Job drawing, mm, ordinate dimensions from the low corner. One solid piece. A direction names the side the tool comes from. Give positions to 0.01 mm unless a question says otherwise; leave off trailing zeros. Write each loop counter-clockwise with the first axis right and the second up, starting at its lowest first coordinate (ties: lowest second). Pieces come first, ordered by that corner, then holes. Notation, with made-up numbers: (66.5, -39.5) - (111.5, -39.5) arc R35 ccw to (111.5, -2.5) - close; hole circle Ø4 at (-32, 32). An arc over 180 degrees is marked (long way). Put each result on its own line as item: value. Start each with the question number.
1. Drop a flat-ended pin along its axis: pin 1 (1.5 mm diameter, centred on x = 2.5, z = 2.5, fed in from +Y). Give the stop position or say it passes through.
2. Cut at D-D on x = 0.6. List the corners of the cut face in (y, z).
3. Cut at A-A on y = 11.25. List the corners of the cut face in (x, z) (1 decimal).
4. Cut at C-C on x = 2.3. List the corners of the cut face in (y, z), and give its area (3 significant figures).
5. Tool access for the marked faces 1 and 2: list every direction of +Z, -Z, +X, -X, +Y, -Y with a clear straight run to the whole face (end or side of a thin tool).
6. Wall check: line 1 (Y direction, x = 0.25, z = 6.75); line 2 (X direction, y = 10, z = 11.25); line 3 (Z direction, x = 1, y = 7.25) (1 decimal). Give the ranges that are in metal, low to high.
7. Cut at B-B on z = 3.75. List the corners of the cut face in (x, y).
8. Mould opens along Z. For the marked faces 3, 4 and 5 say: +Z half, -Z half, draft (parallel to the pull), parting line (faces both ways), or undercut.
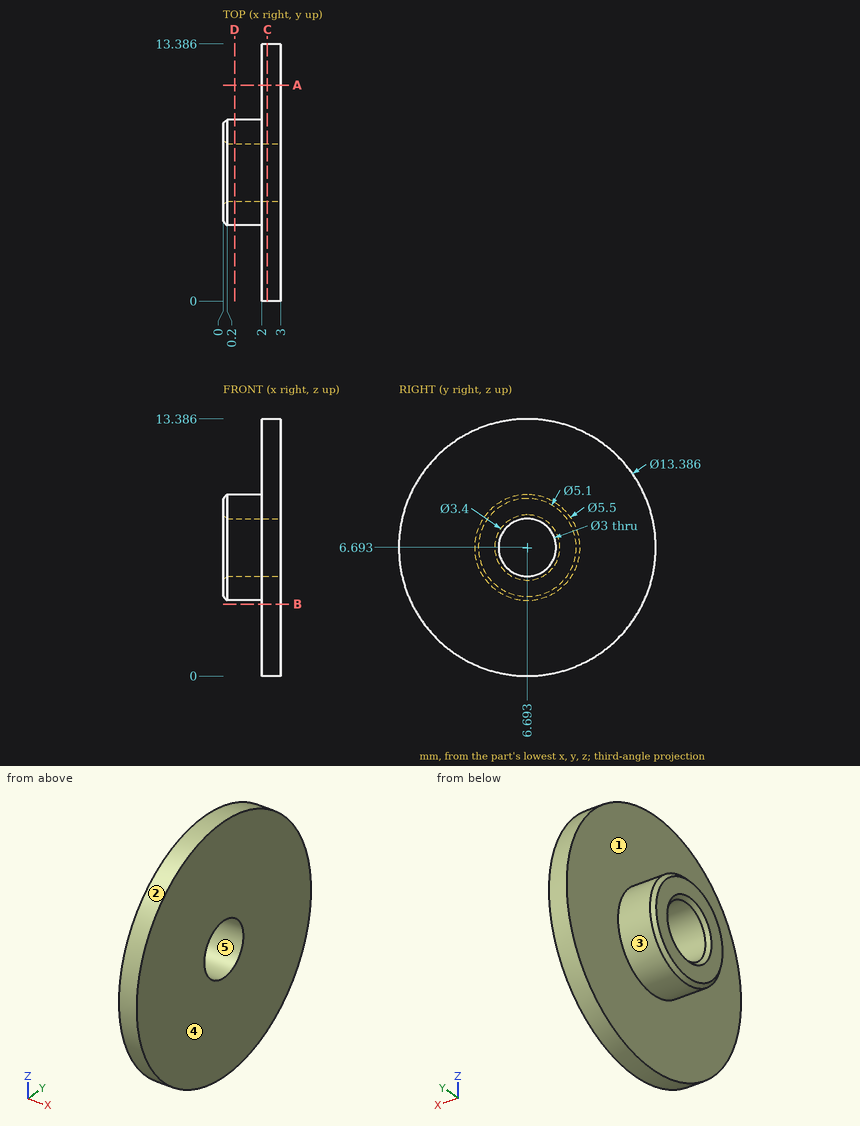
Report:
1. pin 1: stops at y = 12.43
2. outline: circle Ø5.5 at (6.69, 6.69); hole circle Ø3 at (6.69, 6.69)
3. outline: (2, 1.8) - (3, 1.8) - (3, 11.6) - (2, 11.6) - close
4. outline: circle Ø13.39 at (6.69, 6.69); hole circle Ø3 at (6.69, 6.69)
4. area: 134 mm²
5. face 1: -X
5. face 2: +X, -X
6. line 1: y = 3.94 to 5.19, 8.19 to 9.44
6. line 2: x = 2 to 3
6. line 3: z = 4 to 5.3, 8.1 to 9.4
7. outline: (2, 0.68) - (3, 0.68) - (3, 12.7) - (2, 12.7) - close
8. face 3: parting line
8. face 4: draft
8. face 5: undercut
